CAD build for the part. Positions are in the model's coordinates, mm. A direction names the side the tool comes from. Round coordinates to 2 decimals unless told otherwise and drop trailing zeros. Write each loop counter-clockwise with the first axis right and the second up, starting at its lowest first coordinate (ties: lowest second). Pieces come first, ordered by that corner, then holes. Notation, with made-up numbers: (75, -18) -> (88, -18) arc R32 cw to (88, 11) -> close; hole circle Ø3 at (31.5, 68.5). An arc over 180 degrees is marked (long way). Put each result on its own line as item: value. Start each with the question number.
1. 3-axis set-ups, long thin cutter, end or side, ignore diameter. For faces 1 (the flat face through (6.7, 0, 1)), 2 (the cylindrical face through (3.32, 8.46, 2.54)), 3 (the flat face through (-7, -29.45, 1)), 4 (the flat face through (-3.475, -39.24, 5.33)), 5 (the flat face through (5.01, -37, 3)): which of +Z, -Z, +X, -X, +Y, -Y reach the whole face in a straight line?
2. Saw through at C-C on y = -40. List the corners of the cut face in (x, z) (3 decimals).
3. Drill centre lines: line 1 (X direction, y = -32.85, z = 0.5); line 2 (Y direction, x = 7.25, z = 1.05); line 3 (Y direction, x = -3, z = 5.25). Where is each one in solid material? Low to high. Write a range as from..to.
4. Saw through at B-B on x = -7.25. List the corners of the cut face in (y, z).
5. Saw through at A-A on y = -32.85. List the corners of the cut face in (x, z).
6. Flat gauge pins, fed straight in: P1, Ø10, axis at x = 2.5, y = -24, coming from the +Z side; P2, Ø3, axis at x = -3.5, y = -37.5, coming from the +Z side; P3, Ø1.2, axis at y = -1.5, z = 1, coming from the -X side. Where does each tip first touch, or does it go through?
7. Saw through at D-D on z = 2.75. State how many separate pieces and enclosed holes the cut face has, and give its area (3 significant figures).
8. Pull direction X, two halves, no side cores. Call faces 6 (the cylindrical face through (-0.845, -15.307, 6.607)), 7 (the flat face through (0.915, -39.34, 5.33)), 8 (the flat face through (4, 10, 3.55)), 9 (the flat face through (2.525, -24, 1)): pulls with the +X half, pulls with the -X half, needs draft (parallel to the pull), parting line crosses it, or undercut.
from build123d import *

# Parameters (mm, degrees)
SKETCH1_R               = 1.7
BOSS_EXTRUDE1_DEPTH     = 1.55
SKETCH2_R               = 4.5
BOSS_EXTRUDE2_DEPTH     = 2
SKETCH3_R               = 3.9
BOSS_EXTRUDE3_DEPTH     = 9.2
FILLET1_R               = 3
SKETCH4_W               = 2.5
SKETCH4_H               = 2.5
BOSS_EXTRUDE5_DEPTH     = 2.5
CHAMFER1_SIZE           = 0.5
SKETCH5_W               = 0.25
SKETCH5_H               = 1.5
BOSS_EXTRUDE6_DEPTH     = 2
BOSS_EXTRUDE7_START     = -3.8
BOSS_EXTRUDE7_DEPTH     = 0.325
LPATTERN1_START         = 1.55
LPATTERN1_DEPTH         = 2.5
LPATTERN1_START_2       = 5.15
LPATTERN1_2_OUTLINE_W   = 0.65
LPATTERN1_2_OUTLINE_H   = 6.85
LPATTERN1_2_DEPTH       = 0.65
LPATTERN1_START_3       = 4.05
LPATTERN1_3_OUTLINE_W   = 0.65
LPATTERN1_3_OUTLINE_H   = 0.65
LPATTERN1_3_DEPTH       = 1.1
LPATTERN1_4_OUTLINE_W   = 0.02
LPATTERN1_4_OUTLINE_H   = 1.5
LPATTERN1_4_OUTLINE_W_2 = 0.25
LPATTERN1_4_DEPTH       = 2
LPATTERN1_START_4       = -1.605
LPATTERN1_5_DEPTH       = 0.65
LPATTERN1_START_5       = 0.915
LPATTERN1_6_DEPTH       = 0.65
LPATTERN1_START_6       = 3.435
LPATTERN1_7_DEPTH       = 0.65
DELETEFACE1_START       = 5.01
DELETEFACE1_OUTLINE_W   = 1.5
DELETEFACE1_OUTLINE_H   = 2
DELETEFACE1_DEPTH       = 0.25


with BuildPart() as part:
    # Sketch1 → Boss-Extrude1 (new body)
    with BuildSketch(Plane.XY):
        Polygon((-6.7, 17.75), (6.7, 17.75), (6.7, -17.75), (2.525, -17.75), (2.525, -29.45), (10.65, -29.45), (10.65, -37.95), (-10.65, -37.95), (-10.65, -29.45), (-2.525, -29.45), (-2.525, -17.75), (-6.7, -17.75), align=None)
        with Locations(Location((-7.25, -32.85, 0), (0, 0, 180))):
            Circle(SKETCH1_R, mode=Mode.SUBTRACT)
        with Locations(Location((7.25, -32.85, 0), (0, 0, 180))):
            Circle(SKETCH1_R, mode=Mode.SUBTRACT)
    extrude(amount=BOSS_EXTRUDE1_DEPTH)

    # Sketch2 → Boss-Extrude2 (add)
    with BuildSketch(Plane.XY.offset(1.55)):
        with Locations(Location((0, 11.5, 0), (0, 0, 180))):
            Circle(SKETCH2_R)
        with Locations(Location((0, 0, 0), (0, 0, 180))):
            Circle(SKETCH2_R)
        with Locations(Location((0, -11.5, 0), (0, 0, 180))):
            Circle(SKETCH2_R)
    extrude(amount=BOSS_EXTRUDE2_DEPTH)

    # Sketch3 → Boss-Extrude3 (add)
    with BuildSketch(Plane.XY.offset(3.55)):
        Circle(SKETCH3_R)
        with Locations((0, 11.5)):
            Circle(SKETCH3_R)
        with Locations((0, -11.5)):
            Circle(SKETCH3_R)
    extrude(amount=BOSS_EXTRUDE3_DEPTH)

    # Fillet1
    fillet1_edges = [part.edges().sort_by_distance(p)[0] for p in [
        (-3.9, 0, 12.75),
        (-3.9, 11.5, 12.75),
        (-3.9, -11.5, 12.75),
    ]]
    fillet(fillet1_edges, radius=FILLET1_R)

    # Sketch4 → Boss-Extrude5 (add)
    with BuildSketch(Plane.XY.offset(1.55)):
        with Locations((-3.8, -36.7)):
            Rectangle(SKETCH4_W, SKETCH4_H)
    extrude(amount=BOSS_EXTRUDE5_DEPTH)

    # Chamfer1
    chamfer1_edges = [part.edges().sort_by_distance(p)[0] for p in [
        (-2.55, -37.95, 2.8),
        (-2.55, -35.45, 2.8),
        (-5.05, -35.45, 2.8),
        (-5.05, -37.95, 2.8),
    ]]
    chamfer(chamfer1_edges, length=CHAMFER1_SIZE)

    # Sketch5 → Boss-Extrude6 (add)
    with BuildSketch(Plane.XY.offset(1.55)):
        with Locations((-2.425, -36.7)):
            Rectangle(SKETCH5_W, SKETCH5_H)
    extrude(amount=BOSS_EXTRUDE6_DEPTH)

    # Sketch6 → Boss-Extrude7 (add, symmetric)
    with BuildSketch(Plane(origin=(0, 0, 0), x_dir=(0, 0, -1), z_dir=(1, 0, 0)).offset(BOSS_EXTRUDE7_START)):
        with BuildLine():
            Line((-4.05, -36.375), (-5.15, -36.375))
            ThreePointArc((-5.15, -36.375), (-5.609619408, -36.565380592), (-5.8, -37.025))
            Line((-5.8, -37.025), (-5.8, -43.875))
            Line((-5.8, -43.875), (-5.15, -43.875))
            Line((-5.15, -43.875), (-5.15, -37.025))
            Line((-5.15, -37.025), (-4.05, -37.025))
            Line((-4.05, -37.025), (-4.05, -36.375))
        make_face()
    extrude(amount=BOSS_EXTRUDE7_DEPTH, both=True)

    # LPattern1: read off the stored shape, not the designer's step
    # LPattern1 outline → LPattern1 (add)
    with BuildSketch(Plane.XY.offset(LPATTERN1_START)):
        Polygon((-0.01, -35.95), (-0.01, -37.45), (0.49, -37.95), (1.99, -37.95), (2.49, -37.45), (2.49, -35.95), (1.99, -35.45), (0.49, -35.45), align=None)
        Polygon((-0.53, -37.95), (-0.03, -37.45), (-0.03, -35.95), (-0.53, -35.45), (-2.03, -35.45), (-2.53, -35.95), (-2.53, -37.45), (-2.03, -37.95), align=None)
        Polygon((3.01, -35.45), (2.51, -35.95), (2.51, -37.45), (3.01, -37.95), (4.51, -37.95), (5.01, -37.45), (5.01, -35.95), (4.51, -35.45), align=None)
    extrude(amount=LPATTERN1_DEPTH)



with BuildPart() as body_2:
    # LPattern1 2 outline → LPattern1 2 (new body)
    with BuildSketch(Plane.XY.offset(LPATTERN1_START_2)):
        with Locations((1.24, -40.45)):
            Rectangle(LPATTERN1_2_OUTLINE_W, LPATTERN1_2_OUTLINE_H)
        with Locations((-1.28, -40.45)):
            Rectangle(LPATTERN1_2_OUTLINE_W, LPATTERN1_2_OUTLINE_H)
        with Locations((3.76, -40.45)):
            Rectangle(LPATTERN1_2_OUTLINE_W, LPATTERN1_2_OUTLINE_H)
    extrude(amount=LPATTERN1_2_DEPTH)


with BuildPart() as part_1:
    add(part.part)

    add(body_2.part)  # LPattern1 3 merges body 2
    # LPattern1 3 outline → LPattern1 3 (add)
    with BuildSketch(Plane.XY.offset(LPATTERN1_START_3)):
        with Locations((1.24, -36.7)):
            Rectangle(LPATTERN1_3_OUTLINE_W, LPATTERN1_3_OUTLINE_H)
        with Locations((-1.28, -36.7)):
            Rectangle(LPATTERN1_3_OUTLINE_W, LPATTERN1_3_OUTLINE_H)
        with Locations((3.76, -36.7)):
            Rectangle(LPATTERN1_3_OUTLINE_W, LPATTERN1_3_OUTLINE_H)
    extrude(amount=LPATTERN1_3_DEPTH)

    # LPattern1 4 outline → LPattern1 4 (add)
    with BuildSketch(Plane.XY.offset(LPATTERN1_START)):
        with Locations((-0.02, -36.7)):
            Rectangle(LPATTERN1_4_OUTLINE_W, LPATTERN1_4_OUTLINE_H)
        with Locations((2.5, -36.7)):
            Rectangle(LPATTERN1_4_OUTLINE_W, LPATTERN1_4_OUTLINE_H)
        with Locations((5.135, -36.7)):
            Rectangle(LPATTERN1_4_OUTLINE_W_2, LPATTERN1_4_OUTLINE_H)
    extrude(amount=LPATTERN1_4_DEPTH)

    # LPattern1 5 outline → LPattern1 5 (add)
    with BuildSketch(Plane.YZ.offset(LPATTERN1_START_4)):
        with BuildLine():
            ThreePointArc((-36.375, 5.15), (-36.565380592, 5.609619408), (-37.025, 5.8))
            Line((-37.025, 5.8), (-37.025, 5.15))
            Line((-37.025, 5.15), (-36.375, 5.15))
        make_face()
    extrude(amount=LPATTERN1_5_DEPTH)

    # LPattern1 6 outline → LPattern1 6 (add)
    with BuildSketch(Plane.YZ.offset(LPATTERN1_START_5)):
        with BuildLine():
            ThreePointArc((-36.375, 5.15), (-36.565380592, 5.609619408), (-37.025, 5.8))
            Line((-37.025, 5.8), (-37.025, 5.15))
            Line((-37.025, 5.15), (-36.375, 5.15))
        make_face()
    extrude(amount=LPATTERN1_6_DEPTH)

    # LPattern1 7 outline → LPattern1 7 (add)
    with BuildSketch(Plane.YZ.offset(LPATTERN1_START_6)):
        with BuildLine():
            ThreePointArc((-36.375, 5.15), (-36.565380592, 5.609619408), (-37.025, 5.8))
            Line((-37.025, 5.8), (-37.025, 5.15))
            Line((-37.025, 5.15), (-36.375, 5.15))
        make_face()
    extrude(amount=LPATTERN1_7_DEPTH)

    # DeleteFace1: read off the stored shape, not the designer's step
    # DeleteFace1 outline → DeleteFace1 (cut)
    with BuildSketch(Plane.YZ.offset(DELETEFACE1_START)):
        with Locations((-36.7, 2.55)):
            Rectangle(DELETEFACE1_OUTLINE_W, DELETEFACE1_OUTLINE_H)
    extrude(amount=DELETEFACE1_DEPTH, mode=Mode.SUBTRACT)


solid = part_1.part
Return value:
1. face 1: +Z, -Z, +X, +Y
1. face 2: +Z
1. face 3: +Z, -Z, -X
1. face 4: +Z, -Y
1. face 5: +Z, +X, +Y, -Y
2. outline: (-4.125, 5.15) -> (-3.475, 5.15) -> (-3.475, 5.8) -> (-4.125, 5.8) -> close; (-1.605, 5.15) -> (-0.955, 5.15) -> (-0.955, 5.8) -> (-1.605, 5.8) -> close; (0.915, 5.15) -> (1.565, 5.15) -> (1.565, 5.8) -> (0.915, 5.8) -> close; (3.435, 5.15) -> (4.085, 5.15) -> (4.085, 5.8) -> (3.435, 5.8) -> close
3. line 1: x = -10.65..-8.95, -5.55..5.55, 8.95..10.65
3. line 2: y = -37.95..-34.55, -31.15..-29.45
3. line 3: y = -13.99..-9.01, -2.49..2.49, 9.01..13.99
4. outline: (-37.95, 0) -> (-34.55, 0) -> (-34.55, 1.55) -> (-37.95, 1.55) -> close; (-31.15, 0) -> (-29.45, 0) -> (-29.45, 1.55) -> (-31.15, 1.55) -> close
5. outline: (-10.65, 0) -> (-8.95, 0) -> (-8.95, 1.55) -> (-10.65, 1.55) -> close; (-5.55, 0) -> (5.55, 0) -> (5.55, 1.55) -> (-5.55, 1.55) -> close; (8.95, 0) -> (10.65, 0) -> (10.65, 1.55) -> (8.95, 1.55) -> close
6. P1: stops at z = 1.55
6. P2: stops at z = 5.8
6. P3: stops at x = -6.7
7. separate pieces: 4
7. enclosed holes: 0
7. area: 214 mm^2
8. face 6: parting line crosses it
8. face 7: undercut
8. face 8: needs draft
8. face 9: pulls with the +X half
